Autodesk Inventor part; units mm, degrees
ref_plane "YZ Plane" through (0, 0, 0) normal (1, 0, 0) x (0, 1, 0)
ref_plane "XZ Plane" through (0, 0, 0) normal (0, 1, 0) x (-1, 0, 0)
ref_plane "XY Plane" through (0, 0, 0) normal (0, 0, 1) x (1, 0, 0)
sketch "Sketch1" plane through (0, 0, 0) normal (0, 1, 0) x (-1, 0, 0)
  line L0 (0, 279.3478) -> (-39.1304, 279.3478)
  line L1 (-39.1304, 279.3478) -> (-39.1304, -195.6522)
  line L2 (-39.1304, -195.6522) -> (0, -195.6522)
  line L3 (0, -195.6522) -> (0, 279.3478)
  line L4 (-39.1304, 279.3478) -> (-29.1304, 279.3478)
  line L5 (-29.1304, 254.3478) -> (-39.1304, 254.3478)
  line L6 (-39.1304, 254.3478) -> (-39.1304, 279.3478)
  line L7 (-39.1304, -195.6522) -> (-29.1304, -195.6522)
  line L8 (-29.1304, -170.6522) -> (-39.1304, -170.6522)
  line L9 (-39.1304, -170.6522) -> (-39.1304, -195.6522)
  point P0 (0, 0)
  point P1 (-39.1304, 254.3478)
  dimension "d0" = 475
  dimension "d4" = 25
  dimension "d5" = 25
extrude "Extrusion1" add sketch "Sketch1" along normal blind 160
sketch "Sketch2" plane through (0, 0, 279.3478) normal (0, 0, 1) x (1, 0, 0)
  line L0 (0, 160) -> (39.1304, 160)
  line L1 (0, 160) -> (39.1304, 160)
  line L2 (39.1304, 160) -> (39.1304, 0)
  line L3 (39.1304, 0) -> (0, 0)
  line L4 (0, 0) -> (0, 160)
  line L5 (39.1304, 160) -> (29.1304, 160)
  line L6 (29.1304, 160) -> (29.1304, 115)
  line L7 (29.1304, 115) -> (39.1304, 115)
  line L8 (39.1304, 115) -> (39.1304, 160)
  line L9 (39.1304, 0) -> (29.1304, 0)
  line L10 (29.1304, 0) -> (29.1304, 45)
  line L11 (29.1304, 45) -> (39.1304, 45)
  line L12 (39.1304, 45) -> (39.1304, 0)
  circle A0 centre (39.1304, 80) radius 18
  line L13 (35.1304, 75) -> (39.1304, 75)
  line L14 (39.1304, 75) -> (39.1304, 98)
  line L15 (39.1304, 98) -> (35.1304, 98)
  line L16 (35.1304, 98) -> (35.1304, 75)
  line L17 (35.1304, 75) -> (39.1304, 75)
  line L18 (39.1304, 75) -> (39.1304, 62)
  line L19 (39.1304, 62) -> (35.1304, 62)
  line L20 (35.1304, 62) -> (35.1304, 75)
  line L21 (39.1304, 0) -> (39.1304, 160)
  line L22 (0, 160) -> (19.1304, 160)
  line L23 (19.1304, 160) -> (19.1304, 0)
  line L24 (19.1304, 0) -> (0, 0)
  line L25 (0, 0) -> (0, 160)
  point P0 (0, 0)
  point P1 (34.1304, 115)
  point P2 (34.1304, 160)
  point P3 (39.1304, 45)
  point P4 (39.1304, 115)
  dimension "d6" = 10
  dimension "d7" = 45
  dimension "d8" = 45
  dimension "d9" = 4
  dimension "d10" = 36
  dimension "d11" = 80
  dimension "d12" = 80
  dimension "d15" = 20
extrude "Extrusion2" cut sketch "Sketch2" against normal up to surface (475 mm away) contours L0 L23 L3 L4 | L0 L2 L7 L6 | L10 L11 L2 L3 | L2 L13 L16 A0 | A0 L16 L15 | L2 A0 L20 L13 | L19 L20 A0
sketch "Sketch3" plane through (0, 160, 0) normal (0, 1, 0) x (1, 0, 0)
  line L0 (-18, 219) -> (160, 219)
  line L1 (160, 219) -> (160, 60.6522)
  line L2 (160, 60.6522) -> (-18, 60.6522)
  line L3 (-18, 60.6522) -> (-18, 219)
  line L4 (19.1304, -279.3478) -> (29.1304, -279.3478)
  point P0 (0, 0)
  dimension "d16" = 340
extrude "Extrusion3" cut sketch "Sketch3" against normal blind 200
sketch "Sketch4" plane through (39.1304, 98, 279.3478) normal (1, 0, 0) x (0, 0, -1)
  line L0 (340, 0) -> (340, 17)
  line L1 (340, 17) -> (0, 17)
  line L2 (0, 0) -> (0, 17)
  line L3 (0, 0) -> (340, 0)
  line L4 (340, -53) -> (340, -36)
  line L5 (340, -36) -> (0, -36)
  line L6 (0, -53) -> (0, -36)
  line L7 (0, -53) -> (340, -53)
  point P0 (279.3478, -98)
extrude "Extrusion4" add sketch "Sketch4" along normal blind 30
sketch "Sketch5" plane through (19.1304, 0, 279.3478) normal (-1, 0, 0) x (0, 0, 1)
  line L0 (-340, 160) -> (-340, 0)
  line L1 (0, 0) -> (-340, 0)
  line L2 (0, 160) -> (0, 0)
  line L3 (-340, 160) -> (0, 160)
  point P0 (-279.3478, 0)
extrude "Extrusion5" add sketch "Sketch5" along normal blind 5
sketch "Sketch6" plane through (29.1304, 115, 279.3478) normal (0, 0, 1) x (1, 0, 0)
  line L0 (9, 13) -> (-3, 13)
  line L1 (-3, 13) -> (-3, 45)
  line L2 (-3, 45) -> (9, 45)
  line L3 (9, 45) -> (9, 13)
  line L4 (-15, -115) -> (0, -115)
  line L5 (11, -83) -> (-3, -83)
  line L6 (-3, -83) -> (-3, -115)
  line L7 (-3, -115) -> (11, -115)
  line L8 (11, -115) -> (11, -83)
  line L9 (0, -70) -> (40, -70)
  line L10 (0, 0) -> (40, 0)
  line L11 (0, 0) -> (0, 45)
  point P0 (-29.1304, -115)
  point P1 (0, -115)
  dimension "d23" = 13
  dimension "d24" = 13
  dimension "d25" = 3
extrude "Extrusion6" cut sketch "Sketch6" against normal blind 500
sketch "Sketch7" plane through (35.1304, 62, 279.3478) normal (0, 0, 1) x (1, 0, 0)
  line L0 (55, 54) -> (-8, 54)
  line L1 (-8, 54) -> (-8, -18)
  line L2 (-8, -18) -> (55, -18)
  line L3 (55, -18) -> (55, 54)
  line L4 (-6, 53) -> (34, 53)
  line L5 (-6, -17) -> (34, -17)
  line L6 (-6, -30) -> (-6, -17)
  point P0 (-35.1304, -62)
  dimension "d28" = 1
  dimension "d29" = 1
  dimension "d30" = 2
properties part number "MainRails" material "Aluminum 6061"
Check sheet for the modelled part. Datum: model origin and axes. Units: mm. A direction names the side the tool comes from. Round coordinates to 2 decimals unless told otherwise and drop trailing zeros. Order: outer loops, then holes, each group sorted by start corner. A loop starts at its lowest first (then second) coordinate and runs counter-clockwise, first axis right, second up. Notation, with made-up numbers: (53, 15.5) - (57, 15.5) arc R24 cw to (57, 39.5) - close; hole circle Ø5 at (36.5, -3.5). An arc over 180 degrees is marked (long way). Answer as CSV lines item,"result". Start each with the question number.
1) Draft check along Y on faces 1 (the face through (20, 160, 107)), 2 (the face through (35.13, 80, 112)), 3 (the face through (69.13, 54, 112)). Enter one of: +Y half, -Y half, draft (parallel to the pull), parting line (faces both ways), or undercut.
2) Section check C-C (y = 90). Record the cut outline in (x, z).
3) Section check D-D (y = 148.5). Record the cut outline in (x, z), then the cut area to 3 significant figures.
4) Depth check by flat-ended pin: pin 1 (20 mm diameter, centred on x = 48, z = 176.5, fed in from +Y); pin 2 (9.5 mm diameter, centred on y = 148.5, z = 165, fed in from +X); pin 3 (6.5 mm diameter, centred on y = 123, z = 59, fed in from +X). Enter the tip coordinate at first touch or a pass-through.
5) Section check A-A (x = 44). Record the cut outline in (y, z).
6) Scan lines: probe 1 along Y at (x, z) = (66.5, 52.5); probe 2 along Y at (x, z) = (30.5, 185); probe 3 along X at (y, z) = (69.5, 109). Record each from-to range of solid material in increasing order.
7) Section check B-B (z = -1.5). Record the cut outline in (x, y).
8) Tool access check on faces 4 (the face through (52, 62, 112)), 5 (the face through (69.13, 107, 112)), 6 (the face through (26.13, 16, 112)), 7 (the face through (49, 115, 112)). Record the directions out of +Z, -Z, +X, -X, +Y, -Y that give a thin tool (end or side, any length) a straight path to the whole face; none if there is none.
Determined:
1,face 1,"+Y half"
1,face 2,"undercut"
1,face 3,"draft"
2,outline,"(14.13, -60.65) - (35.13, -60.65) - (35.13, 279.35) - (14.13, 279.35) - close"
3,outline,"(14.13, -60.65) - (26.13, -60.65) - (26.13, 279.35) - (14.13, 279.35) - close"
3,area,"4,080 mm^2"
4,pin 1,"y = 115"
4,pin 2,"x = 26.13"
4,pin 3,"x = 29.13"
5,outline,"(45, -60.65) - (62, -60.65) - (62, 279.35) - (45, 279.35) - close; (98, -60.65) - (115, -60.65) - (115, 279.35) - (98, 279.35) - close"
6,probe 1,"45 to 62, 98 to 115"
6,probe 2,"45 to 115"
6,probe 3,"14.13 to 35.13"
7,outline,"(14.13, 0) - (26.13, 0) - (26.13, 32) - (29.13, 32) - (29.13, 45) - (69.13, 45) - (69.13, 62) - (35.13, 62) - (35.13, 98) - (69.13, 98) - (69.13, 115) - (29.13, 115) - (29.13, 128) - (26.13, 128) - (26.13, 160) - (14.13, 160) - close"
8,face 4,"+Z, -Z, +X"
8,face 5,"+Z, -Z, +X, +Y, -Y"
8,face 6,"+Z, -Z, +X, -Y"
8,face 7,"+Z, -Z, +X, +Y"
